Job drawing, mm, ordinate dimensions from the low corner. One solid piece. Round coordinates to 2 decimals unless told otherwise and drop trailing zeros. Order: outer loops, then holes, each group sorted by start corner. A loop starts at its lowest first (then second) coordinate and runs counter-clockwise, first axis right, second up. Notation, with made-up numbers: (-2, -3) - (28, -3) arc R20 cw to (28, 12) - close; hole circle Ø4 at (1.5, 10). An arc over 180 degrees is marked (long way). Use one line per item in the form item = value. Start each with the question number.
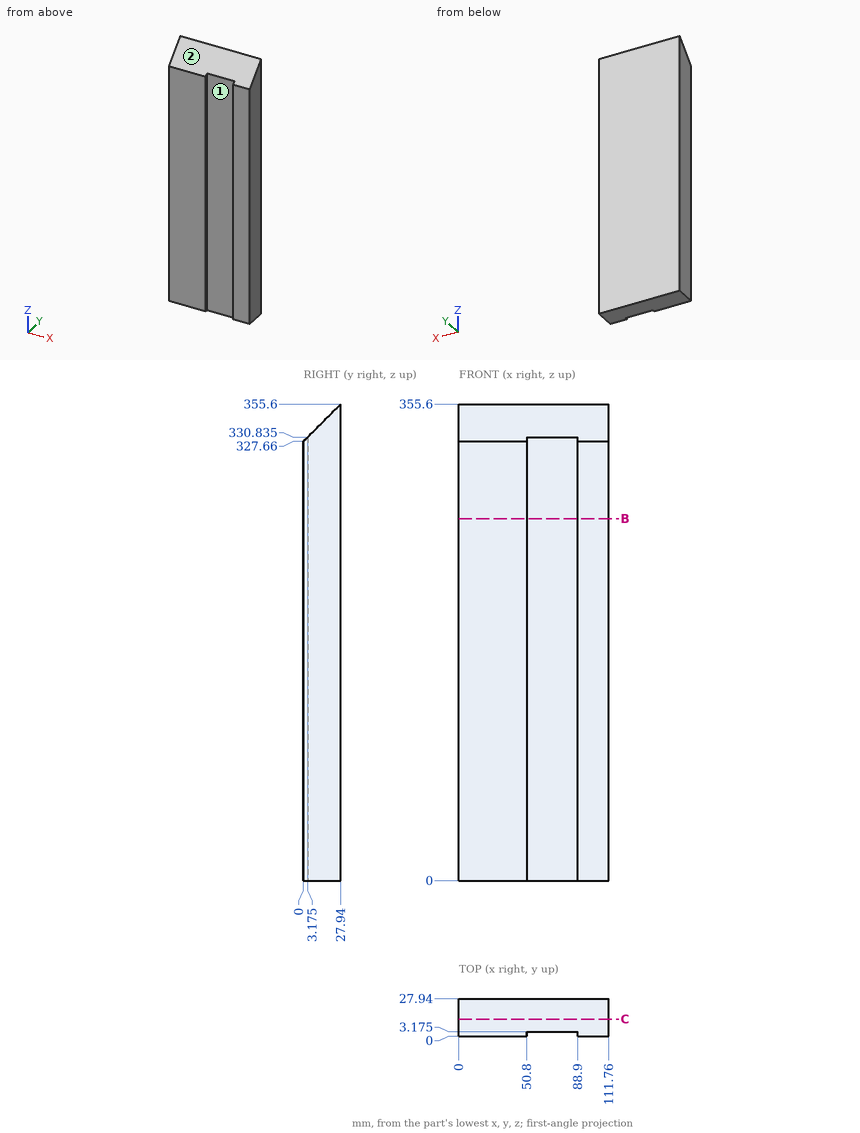
(1) Wall check: line 1 (X direction, y = 2.5, z = 189.5); line 2 (Y direction, x = 63, z = 239) (3 decimals); line 3 (Z direction, x = 86, y = 22.25). Give the ranges that are in metal, low to high. Write a range as [from, to].
(2) Slice it at B-B (z = 270). Give the cut face in (x, y) (3 decimals), and give its area (3 significant figures).
(3) Flat gauge pins, fed straight in: P1, Ø1.5, axis at x = 90, y = 4, coming from the -Z side; P2, Ø4, axis at x = 51, y = 15.5, coming from the +Z side; P3, Ø19, axis at x = 78.5, z = 111, coming from the -Y side (3 decimals). Where does each tip first touch, or does it go through?
(4) Slice it at C-C (y = 12.5). Give the cut face in (x, z).
(5) Mould opens along X. For the marked faces 1 and 2 say: pulls with the +X half, pulls with the -X half, needs draft (parallel to the pull), parting line crosses it, or undercut.
Results list:
q1.line_1 = [0, 50.8], [88.9, 111.76]
q1.line_2 = [3.175, 27.94]
q1.line_3 = [0, 349.91]
q2.outline = (0, 0) - (50.8, 0) - (50.8, 3.175) - (88.9, 3.175) - (88.9, 0) - (111.76, 0) - (111.76, 27.94) - (0, 27.94) - close
q2.area = 3,000 mm²
q3.P1 = 0
q3.P2 = 345.16
q3.P3 = 3.175
q4.outline = (0, 0) - (111.76, 0) - (111.76, 340.16) - (0, 340.16) - close
q5.face_1 = undercut
q5.face_2 = needs draft
